from build123d import *

# Parameters (mm, degrees)
SKETCH1_R                                           = 60
SKETCH1_R_2                                         = 26.3
BOSS_EXTRUDE1_DEPTH                                 = 7
CSK_FOR_M6_COUNTERSUNK_FLAT_HEAD_SCREW1_D           = 6.6
CSK_FOR_M6_COUNTERSUNK_FLAT_HEAD_SCREW1_CSINK_D     = 12.6
CSK_FOR_M6_COUNTERSUNK_FLAT_HEAD_SCREW1_CSINK_ANGLE = 90
CHAMFER1_SIZE                                       = 0.5


with BuildPart() as part:
    # Sketch1 → Boss-Extrude1 (new body)
    with BuildSketch(Plane.XY):
        Circle(SKETCH1_R)
        Circle(SKETCH1_R_2, mode=Mode.SUBTRACT)
    extrude(amount=BOSS_EXTRUDE1_DEPTH)

    # CSK for M6 Countersunk Flat Head Screw1 (through all)
    with Locations(Plane.XY.offset(7)):
        with Locations((-37.123106012, 37.123106012), (0, 52.5), (37.123106012, 37.123106012), (52.5, 0), (37.123106012, -37.123106012), (0, -52.5), (-37.123106012, -37.123106012), (-52.5, 0)):
            CounterSinkHole(CSK_FOR_M6_COUNTERSUNK_FLAT_HEAD_SCREW1_D / 2, CSK_FOR_M6_COUNTERSUNK_FLAT_HEAD_SCREW1_CSINK_D / 2, counter_sink_angle=CSK_FOR_M6_COUNTERSUNK_FLAT_HEAD_SCREW1_CSINK_ANGLE)

    # Chamfer1
    chamfer1_edges = [part.edges().sort_by_distance(p)[0] for p in [
        (-33.823106012, 37.123106012, 0),
        (-60, 0, 0),
        (-49.2, 0, 0),
        (-33.823106012, -37.123106012, 0),
        (3.3, -52.5, 0),
        (40.423106012, -37.123106012, 0),
        (55.8, 0, 0),
        (-60, 0, 7),
        (-26.3, 0, 0),
        (40.423106012, 37.123106012, 0),
        (-26.3, 0, 7),
        (3.3, 52.5, 0),
    ]]
    chamfer(chamfer1_edges, length=CHAMFER1_SIZE)


solid = part.part
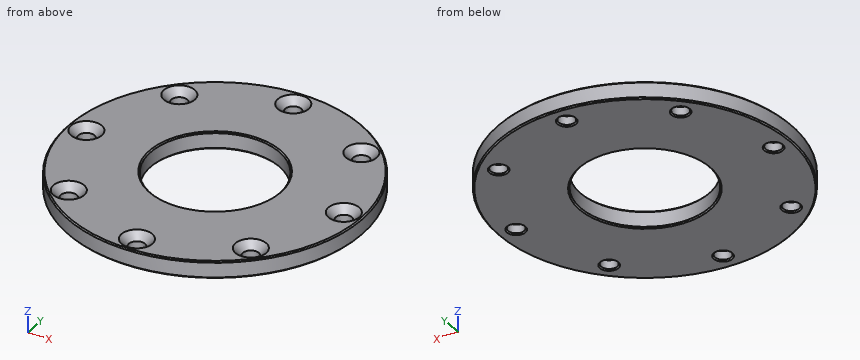
Verification items for the finished model (mm, model axes). Give positions to 0.01 mm unless a question says otherwise; leave off trailing zeros. Use CSV: the item, a comma, the result in double quotes.
(1) Material ranges on L1, parallel to X at y = -2, z = 2; L2, parallel to Y at x = -3, z = 6.75; L3, parallel to Y at x = 4, z = 5.5, recorded low to high.
Derived:
L1,"x = -59.97 to -55.12, -49.88 to -26.22, 26.22 to 49.88, 55.12 to 59.97"
L2,"y = -59.67 to -57.75, -47.25 to -26.38, 26.38 to 47.25, 57.75 to 59.67"
L3,"y = -59.87 to -55.15, -49.85 to -25.99, 25.99 to 49.85, 55.15 to 59.87"
(2) Sectioned sample at A-A (x = 0). Give the number of separate pieces and of enclosed holes in the cut face, plus the area to 3 significant figures.
Derived:
separate pieces,"4"
enclosed holes,"0"
area,"360 mm^2"
(3) Go/stop test with flat-tipped pins: pin 1 (6 mm diameter, centred on x = -52.5, y = 0, fed in from -Z) (3 decimals); pin 2 (8 mm diameter, centred on x = -32.5, y = -19, fed in from -Z); pin 3 (8.5 mm diameter, centred on x = 52.5, y = 0, fed in from +Z); pin 4 (4 mm diameter, centred on x = 12.5, z = 3.5, fed in from +Y). Record where each tip stops, or that it passes through.
Derived:
pin 1,"passes through"
pin 2,"stops at z = 0"
pin 3,"stops at z = 4.95"
pin 4,"stops at y = 59.07"
